The model under review builds one solid part; all positions refer to its coordinate system, in mm. Round coordinates to 2 decimals unless told otherwise and drop trailing zeros. Loops run counter-clockwise (first coordinate to the right, second up) from the corner with the lowest first, then second, coordinate; pieces in that order, holes last. Notation, with made-up numbers: (4.25, 87) -> (59.25, 87) arc R23 cw to (59.25, 95) -> close; hole circle Ø11 at (-32.75, 4.25). An arc over 180 degrees is marked (long way). Use a Markdown table: item, result. Add a question column.
1) Consider section A-A on z = 3.25. Give the boundary of the cut face in (x, y).
2) Wall thickness on probe 1 along Y at (x, z) = (-6.7, 3.25); probe 2 along Z at (x, y) = (-2.75, 34): over which ranges is each line inside the solid? List them lowest first.
3) Consider section C-C on y = 201.5. Give the boundary of the cut face in (x, z).
4) Insertion check: pin 1 (2.5 mm diameter, centred on x = 0, y = 242.5, fed in from -Z). The pin has a flat end and moves straight along its axis. Give the tip position at first contact, or say it passes through.
5) Consider section B-B on y = 113. Give the boundary of the cut face in (x, z), plus the area to 3 significant figures.
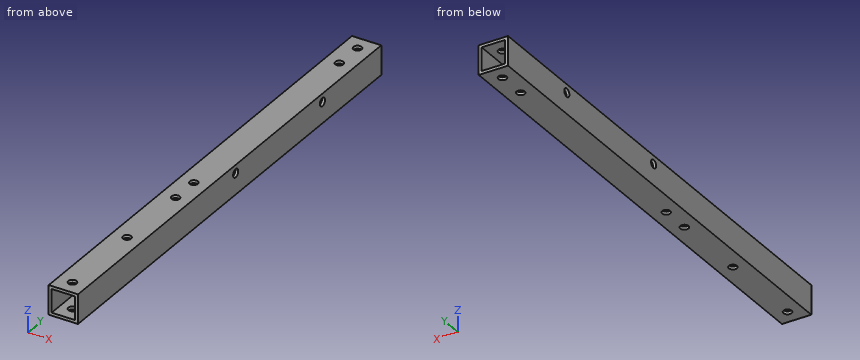
from build123d import *

# Parameters (mm, degrees)
SKETCH_1_W          = 15
SKETCH_1_H          = 15
SKETCH_1_W_2        = 12
SKETCH_1_H_2        = 12
EXTRUDE_1_DEPTH     = 250
SKETCH_2_R          = 2.1
CUT_EXTRUDE_1_DEPTH = 251.561868607
SKETCH_3_R          = 2.1
CUT_EXTRUDE_2_DEPTH = 251.561868607
SKETCH_4_R          = 2.1
CUT_EXTRUDE_3_DEPTH = 251.561868607
SKETCH_5_R          = 2.1
CUT_EXTRUDE_4_DEPTH = 251.561868607


with BuildPart() as part:
    # ｽｹｯﾁ1 → 押し出し-薄板1 (new body)
    with BuildSketch(Plane(origin=(0, 0, 0), x_dir=(1, 0, 0), z_dir=(0, 1, 0))):
        Rectangle(SKETCH_1_W, SKETCH_1_H)
        Rectangle(SKETCH_1_W_2, SKETCH_1_H_2, mode=Mode.SUBTRACT)
    extrude(amount=EXTRUDE_1_DEPTH)

    # ｽｹｯﾁ2 → ｶｯﾄ - 押し出し1 (cut, through all)
    with BuildSketch(Plane.XY.offset(7.5)):
        with Locations((0, 52.5)):
            Circle(SKETCH_2_R)
        with Locations((0, 7.5)):
            Circle(SKETCH_2_R)
    extrude(amount=-CUT_EXTRUDE_1_DEPTH, mode=Mode.SUBTRACT)

    # ｽｹｯﾁ3 → ｶｯﾄ - 押し出し2 (cut, through all)
    with BuildSketch(Plane.XY.offset(7.5)):
        with Locations((0, 107.5)):
            Circle(SKETCH_3_R)
        with Locations((0, 92.5)):
            Circle(SKETCH_3_R)
    extrude(amount=-CUT_EXTRUDE_2_DEPTH, mode=Mode.SUBTRACT)

    # ｽｹｯﾁ4 → ｶｯﾄ - 押し出し3 (cut, through all)
    with BuildSketch(Plane(origin=(7.5, 0, 0), x_dir=(0, 0, -1), z_dir=(1, 0, 0))):
        with Locations((-3.25, 130)):
            Circle(SKETCH_4_R)
        with Locations((-3.25, 201.5)):
            Circle(SKETCH_4_R)
    extrude(amount=-CUT_EXTRUDE_3_DEPTH, mode=Mode.SUBTRACT)

    # ｽｹｯﾁ5 → ｶｯﾄ - 押し出し4 (cut, through all)
    with BuildSketch(Plane.XY.offset(7.5)):
        with Locations((0, 227.5)):
            Circle(SKETCH_5_R)
        with Locations((0, 242.5)):
            Circle(SKETCH_5_R)
    extrude(amount=-CUT_EXTRUDE_4_DEPTH, mode=Mode.SUBTRACT)


solid = part.part
Result set:
| question | item | result |
|---|---|---|
| 1 | outline | (-7.5, 0) -> (-6, 0) -> (-6, 127.9) -> (-7.5, 127.9) -> close; (-7.5, 132.1) -> (-6, 132.1) -> (-6, 199.4) -> (-7.5, 199.4) -> close; (-7.5, 203.6) -> (-6, 203.6) -> (-6, 250) -> (-7.5, 250) -> close; (6, 0) -> (7.5, 0) -> (7.5, 127.9) -> (6, 127.9) -> close; (6, 132.1) -> (7.5, 132.1) -> (7.5, 199.4) -> (6, 199.4) -> close; (6, 203.6) -> (7.5, 203.6) -> (7.5, 250) -> (6, 250) -> close |
| 2 | probe 1 | 0 to 127.9, 132.1 to 199.4, 203.6 to 250 |
| 2 | probe 2 | -7.5 to -6, 6 to 7.5 |
| 3 | outline | (-7.5, -7.5) -> (7.5, -7.5) -> (7.5, 1.15) -> (6, 1.15) -> (6, -6) -> (-6, -6) -> (-6, 1.15) -> (-7.5, 1.15) -> close; (-7.5, 5.35) -> (-6, 5.35) -> (-6, 6) -> (6, 6) -> (6, 5.35) -> (7.5, 5.35) -> (7.5, 7.5) -> (-7.5, 7.5) -> close |
| 4 | pin 1 | through |
| 5 | outline | (-7.5, -7.5) -> (7.5, -7.5) -> (7.5, 7.5) -> (-7.5, 7.5) -> close; hole (-6, -6) -> (6, -6) -> (6, 6) -> (-6, 6) -> close |
| 5 | area | 81.0 mm2 |
